Here's how the part is built. I have some questions about the finished solid (model axes, mm). Face numbers are marked on the shaded views. A direction names the side the tool comes from. Give positions to 0.01 mm unless a question says otherwise; leave off trailing zeros. Loops run counter-clockwise (first coordinate to the right, second up) from the corner with the lowest first, then second, coordinate; pieces in that order, holes last.
Q1. If we section it at A-A (z = -12.5): Please give me the cut outline in (x, y).
Q2. Will these pins go through, and if not, where does the flat tip stop? P1, Ø5, axis at x = 31.5, z = 13.5, coming from the +Y side; P2, Ø1, axis at x = 31, z = 6, coming from the +Y side; P3, Ø6, axis at x = -7, z = -5, coming from the -Y side; P4, Ø2, axis at x = -10.5, y = 119.5, coming from the -Z side.
Q3. We'd pull the mould along X, two halves only. Please class the marked faces 1, 2 and 3: +X half, -X half, draft (parallel to the pull), parting line (faces both ways), or undercut.
Q4. I need wall thicknesses on line 1 (X direction, y = 14.5, z = -12.5); line 2 (X direction, y = 4, z = -12.5); line 3 (Y direction, x = -9, z = -9). Which ranges of each line are inside material? Lowest first, please.
Q5. If we section it at B-B (y = 88.5): Please give me the cut outline in (x, z), plus the area to 3 significant figures.
Q6. For the marked faces 4, 5, 6 and 7, which set-ups out of +Z, -Z, +X, -X, +Y, -Y let a thin tool reach every point of the face, with its end or its side?
Q7. If we section it at C-C (x = 0): Please give me the cut outline in (y, z) (3 decimals), plus the area to 3 significant figures.
from build123d import *

# Parameters (mm, degrees)
BOSS_EXTRUDE1_DEPTH = 20
BOSS_EXTRUDE2_DEPTH = 160
SKETCH3_R           = 58
CUT_EXTRUDE1_DEPTH  = 50
SKETCH4_R           = 3
CUT_EXTRUDE2_DEPTH  = 4
CIRPATTERN1_COUNT   = 3
BOSS_EXTRUDE3_DEPTH = 20
SKETCH5_R           = 3.2
CUT_EXTRUDE3_DEPTH  = 190.835375153
FILLET1_R           = 10
FILLET2_R           = 5
FILLET4_R           = 0.5
SKETCH7_R           = 5.25
CUT_EXTRUDE4_DEPTH  = 10


with BuildPart() as part:
    # Sketch1 → Boss-Extrude1 (new body)
    with BuildSketch(Plane(origin=(0, 0, 0), x_dir=(1, 0, 0), z_dir=(0, 1, 0))):
        with BuildLine():
            Line((-10, 0), (-10, 74.330343737))
            ThreePointArc((-10, 74.330343737), (0, 75), (10, 74.330343737))
            Line((10, 74.330343737), (10, 0))
            ThreePointArc((10, 0), (0, -10), (-10, 0))
        make_face()
    boss_extrude1 = extrude(amount=BOSS_EXTRUDE1_DEPTH)

    # Sketch2 → Boss-Extrude2 (add)
    with BuildSketch(Plane(origin=(0, 20, 0), x_dir=(1, 0, 0), z_dir=(0, 1, 0))):
        with BuildLine():
            Line((-10, 74.330343737), (-10, 38.729833462))
            ThreePointArc((-10, 38.729833462), (0, 40), (10, 38.729833462))
            Line((10, 38.729833462), (10, 74.330343737))
            ThreePointArc((10, 74.330343737), (0, 75), (-10, 74.330343737))
        make_face()
    boss_extrude2 = extrude(amount=BOSS_EXTRUDE2_DEPTH)

    # Sketch3 → Cut-Extrude1 (cut)
    with BuildSketch(Plane(origin=(0, 180, 0), x_dir=(1, 0, 0), z_dir=(0, 1, 0))):
        Circle(SKETCH3_R)
    cut_extrude1 = extrude(amount=-CUT_EXTRUDE1_DEPTH, mode=Mode.SUBTRACT)

    # Sketch4 → Cut-Extrude2 (cut)
    with BuildSketch(Plane(origin=(0, 130, 0), x_dir=(1, 0, 0), z_dir=(0, 1, 0))):
        with Locations(Location((0, 53.975, 0), (0, 0, 270))):
            Circle(SKETCH4_R)
    cut_extrude2 = extrude(amount=-CUT_EXTRUDE2_DEPTH, mode=Mode.SUBTRACT)

    # CirPattern1: Boss-Extrude1, Boss-Extrude2, Cut-Extrude1, Cut-Extrude2 ×3 about axis
    cirpattern1_axis = Axis((0, 0, 0), (0, 1, 0))
    add([boss_extrude1.rotate(cirpattern1_axis, i * 360 / CIRPATTERN1_COUNT) for i in range(1, CIRPATTERN1_COUNT)])
    add([boss_extrude2.rotate(cirpattern1_axis, i * 360 / CIRPATTERN1_COUNT) for i in range(1, CIRPATTERN1_COUNT)])
    add([cut_extrude1.rotate(cirpattern1_axis, i * 360 / CIRPATTERN1_COUNT) for i in range(1, CIRPATTERN1_COUNT)], mode=Mode.SUBTRACT)
    add([cut_extrude2.rotate(cirpattern1_axis, i * 360 / CIRPATTERN1_COUNT) for i in range(1, CIRPATTERN1_COUNT)], mode=Mode.SUBTRACT)

    # Sketch6 → Boss-Extrude3 (add)
    with BuildSketch(Plane(origin=(0, 0, 0), x_dir=(1, 0, 0), z_dir=(0, 1, 0))):
        with BuildLine():
            Line((15, -20), (-15, -20))
            ThreePointArc((-15, -20), (-18.535533906, -18.535533906), (-20, -15))
            Line((-20, -15), (-20, 15))
            ThreePointArc((-20, 15), (-18.535533906, 18.535533906), (-15, 20))
            Line((-15, 20), (15, 20))
            ThreePointArc((15, 20), (18.535533906, 18.535533906), (20, 15))
            Line((20, 15), (20, -15))
            ThreePointArc((20, -15), (18.535533906, -18.535533906), (15, -20))
        make_face()
    extrude(amount=BOSS_EXTRUDE3_DEPTH)

    # Sketch5 → Cut-Extrude3 (cut, through all)
    with BuildSketch(Plane(origin=(0, 20, 0), x_dir=(1, 0, 0), z_dir=(0, 1, 0))):
        with Locations(Location((-12.5, 12.5, 0), (0, 0, 270))):
            Circle(SKETCH5_R)
        with Locations(Location((12.5, 12.5, 0), (0, 0, 270))):
            Circle(SKETCH5_R)
        with Locations(Location((-12.5, -12.5, 0), (0, 0, 270))):
            Circle(SKETCH5_R)
        with Locations(Location((12.5, -12.5, 0), (0, 0, 270))):
            Circle(SKETCH5_R)
    extrude(amount=-CUT_EXTRUDE3_DEPTH, mode=Mode.SUBTRACT)

    # Fillet1
    fillet1_edges = [part.edges().sort_by_distance(p)[0] for p in [
        (0, 20, -40),
        (34.641016151, 20, 20),
        (-34.641016151, 20, 20),
    ]]
    fillet(fillet1_edges, radius=FILLET1_R)

    # Fillet2
    fillet2_edges = [part.edges().sort_by_distance(p)[0] for p in [
        (34.641016151, 130, 20),
        (-14.641016151, 10, 20),
        (-20, 10, 0),
        (20, 10, 0),
        (10, 10, -20),
        (-10, 10, -20),
        (14.641016151, 10, 20),
        (0, 130, -40),
        (-34.641016151, 130, 20),
    ]]
    fillet(fillet2_edges, radius=FILLET2_R - 0.0001)  # a hair under: the kernel refuses the full size

    # Fillet4
    fillet4_edges = [part.edges().sort_by_distance(p)[0] for p in [
        (50.229473419, 130, 29),
        (-50.229473419, 130, 29),
        (0, 130, -58),
    ]]
    fillet(fillet4_edges, radius=FILLET4_R)

    # Sketch7 → Cut-Extrude4 (cut)
    with BuildSketch(Plane(origin=(0, 20, 0), x_dir=(1, 0, 0), z_dir=(0, 1, 0))):
        with Locations(Location((-12.5, 12.5, 0), (0, 0, 270))):
            Circle(SKETCH7_R)
        with Locations(Location((12.5, 12.5, 0), (0, 0, 270))):
            Circle(SKETCH7_R)
        with Locations(Location((12.5, -12.5, 0), (0, 0, 270))):
            Circle(SKETCH7_R)
        with Locations(Location((-12.5, -12.5, 0), (0, 0, 270))):
            Circle(SKETCH7_R)
    extrude(amount=-CUT_EXTRUDE4_DEPTH, mode=Mode.SUBTRACT)


solid = part.part
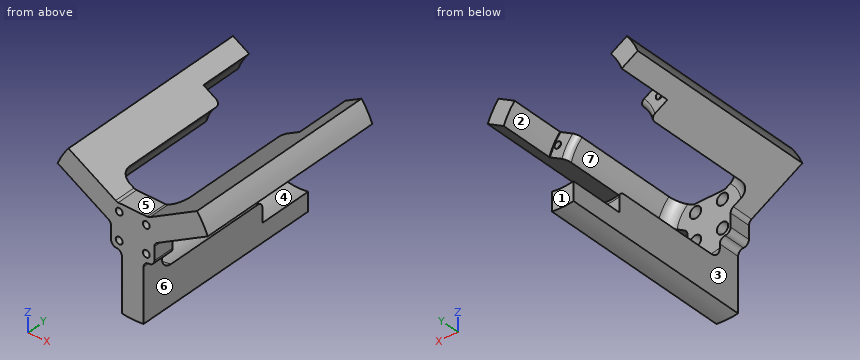
Check sheet entries:
1. outline: (-20, 0) - (-15.7, 0) - (-15.7, 10) - (-17.75, 10) - (-17.75, 20) - (-20, 20) - close; (-9.3, 0) - (9.3, 0) - (9.3, 10) - (7.25, 10) - (7.25, 20) - (-7.25, 20) - (-7.25, 10) - (-9.3, 10) - close; (15.7, 0) - (20, 0) - (20, 20) - (17.75, 20) - (17.75, 10) - (15.7, 10) - close
2. P1: stops at y = 22.64
2. P2: stops at y = 20.17
2. P3: stops at y = 0
2. P4: stops at z = -74.4
3. face 1: draft
3. face 2: undercut
3. face 3: -X half
4. line 1: x = -20 to -17.75, -7.25 to 7.25, 17.75 to 20
4. line 2: x = -20 to -15.7, -9.3 to 9.3, 15.7 to 20
4. line 3: y = 0 to 10
5. outline: (-69.37, 28.5) - (-38.54, 10.7) arc R40 cw to (-28.54, 28.03) - (-59.37, 45.83) arc R75 ccw to start; (-10, -74.33) arc R75 ccw to (10, -74.33) - (10, -38.73) arc R40 cw to (-10, -38.73) - close; (28.54, 28.03) arc R40 cw to (38.54, 10.7) - (69.37, 28.5) arc R75 ccw to (59.37, 45.83) - close
5. area: 2,110 mm2
6. face 4: +Z, +Y
6. face 5: +Z, +Y, -Y
6. face 6: -Z, +X, +Y, -Y
6. face 7: -Z, +Y
7. outline: (0, -75) - (180, -75) - (180, -58) - (130.5, -58) arc R0.5 cw to (130, -57.5) - (130, -56.975) - (126, -56.975) - (126, -50.975) - (130, -50.975) - (130, -45) arc R5 ccw to (125, -40) - (30, -40) arc R10 cw to (20, -30) - (20, 20) - (0, 20) - close
7. area: 6,590 mm2
